Check sheet for the modelled part. Datum: model origin and axes. Units: mm. Face numbers are marked on the shaded views. Give positions to 0.01 mm unless a question says otherwise; leave off trailing zeros. Order: outer loops, then holes, each group sorted by start corner. A loop starts at its lowest first (then second) coordinate and runs counter-clockwise, first axis right, second up. Notation, with made-up numbers: (-19, 26) -> (32, 26) arc R20 cw to (32, 56) -> close; hole circle Ø5 at (63, 40). An arc over 180 degrees is marked (long way). Answer in a Markdown table with one row per item. Add a question column.
(1) Thickness scan on L1, parallel to Z at x = -27, y = 0; L2, parallel to X at y = 4.5, z = 0.75; L3, parallel to Z at x = -21, y = -6. Record the ranges inside material, lowest first. Write a range as [from, to].
(2) Cross-section at A-A (x = -26). Record the cut outline in (y, z).
(3) Release check for a two-part mould opening along Z. For the marked faces 1, 2 and 3 record: released by +Z, released by -Z, zero draft, split by the parting line, or undercut.
(4) Go/stop test with flat-tipped pins: pin 1 (1 mm diameter, centred on x = -21, y = -4.5, fed in from +Z); pin 2 (4 mm diameter, centred on x = -25.5, y = -7, fed in from +Z); pin 3 (6 mm diameter, centred on y = 2.5, z = 0, fed in from +X). Record where each tip stops, or that it passes through.
(5) Cross-section at B-B (x = -21.5). Record the cut outline in (y, z).
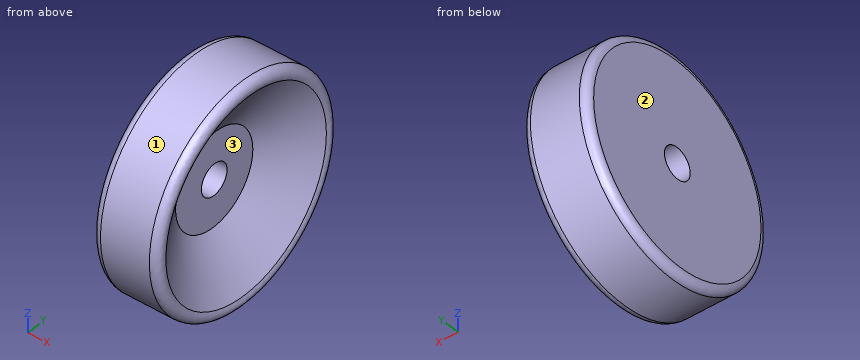
```python
from build123d import *

# Parameters (mm, degrees)
FILLET001_R = 1
FILLET002_R = 1


with BuildPart() as part:
    # Sketch004 → Revolution (revolve)
    with BuildSketch(Plane.XY):
        Polygon((2, 14), (2, 2), (6, 2), (6, 6), (11, 14), align=None)
    revolve(axis=Axis((0, 0, 0), (1, 0, 0)))

    # Fillet001
    fillet001_edges = [part.edges().sort_by_distance(p)[0] for p in [
        (2, -14, 0),
    ]]
    fillet(fillet001_edges, radius=FILLET001_R)

    # Fillet002
    fillet002_edges = [part.edges().sort_by_distance(p)[0] for p in [
        (11, -14, 0),
    ]]
    fillet(fillet002_edges, radius=FILLET002_R)


with BuildPart() as part_1:
    # Body001 placement: moved
    add(part.part.moved(Location((-30, 0, 0))))


solid = part_1.part
```
Answer below:
| question | item | result |
|---|---|---|
| 1 | L1 | z = [-14, -2], [2, 14] |
| 1 | L2 | x = [-28, -24] |
| 1 | L3 | z = [-12.65, -8.98], [8.98, 12.65] |
| 2 | outline | circle Ø28 at (0, 0); hole circle Ø4 at (0, 0) |
| 3 | face 1 | split by the parting line |
| 3 | face 2 | zero draft |
| 3 | face 3 | undercut |
| 4 | pin 1 | stops at z = 13.42 |
| 4 | pin 2 | stops at z = 13.08 |
| 4 | pin 3 | stops at x = -24 |
| 5 | outline | circle Ø28 at (0, 0); hole circle Ø20 at (0, 0) |
